```python
from build123d import *

# Parameters (mm, degrees)
F0_W      = 3
F0_H      = 11
F1_DEPTH  = 15.9
F2_W      = 6
F2_H      = 9
F3_DEPTH  = 31.001
F4_R      = 1
F5_DEPTH  = 6.9
F6_R      = 1.05
F7_DEPTH  = 4
F8_W      = 3
F8_H      = 1
F8_W_2    = 1
F8_H_2    = 3
F9_DEPTH  = 1
F10_R     = 1
F11_DEPTH = 3
F12_W     = 12
F12_H     = 8
F13_DEPTH = 3


with BuildPart() as f1:
    # F0 (on Front) → F1 (new body)
    with BuildSketch(Plane.XZ):
        with Locations((1.5, 8.5)):
            Rectangle(F0_W, F0_H)
        Polygon((3, 3), (0, 3), (0, 0), (31, 0), (31, 3), (28, 3), align=None)
        with Locations((29.5, 8.5)):
            Rectangle(F0_W, F0_H)
    extrude(amount=F1_DEPTH)

    # F2 (on face) → F3 (cut, through all)
    with BuildSketch(Plane.YZ.offset(31)):
        with Locations((-6, 9.5)):
            Rectangle(F2_W, F2_H)
    extrude(amount=-F3_DEPTH, mode=Mode.SUBTRACT)

    # F4 (on face) → F5 (cut, through all)
    with BuildSketch(Plane.XZ.offset(15.9)):
        with Locations((1.7, 8.95)):
            Circle(F4_R)
        with Locations((29.3, 8.95)):
            Circle(F4_R)
    extrude(amount=-F5_DEPTH, mode=Mode.SUBTRACT)

    # F6 (on face) → F7 (cut)
    with BuildSketch(Plane(origin=(0, 0, 0), x_dir=(-1, 0, 0), z_dir=(0, 1, 0))):
        with Locations((-26, 1.5)):
            Circle(F6_R)
        with Locations((-5, 1.5)):
            Circle(F6_R)
    extrude(amount=-F7_DEPTH, mode=Mode.SUBTRACT)

    # F8 (on face) → F9 (join)
    with BuildSketch(Plane(origin=(0, 0, 0), x_dir=(-1, 0, 0), z_dir=(0, 1, 0))):
        with Locations((-20.5, 1.5)):
            Rectangle(F8_W, F8_H)
        with Locations((-10.5, 1.5)):
            Rectangle(F8_W, F8_H)
        with Locations((-29, 9.5)):
            Rectangle(F8_W_2, F8_H_2)
        with Locations((-2, 9.5)):
            Rectangle(F8_W_2, F8_H_2)
    extrude(amount=F9_DEPTH)

    # F10 (on face) → F11 (cut)
    with BuildSketch(Plane.XY.offset(14)):
        with Locations((29.4, -1.5)):
            Circle(F10_R)
        with Locations((1.6, -1.5)):
            Circle(F10_R)
    extrude(amount=-F11_DEPTH, mode=Mode.SUBTRACT)

    # F12 (on face) → F13 (cut, through all)
    with BuildSketch(Plane.XY.offset(3)):
        with Locations((16, -7.9)):
            Rectangle(F12_W, F12_H)
    extrude(amount=-F13_DEPTH, mode=Mode.SUBTRACT)


solid = f1.part
```
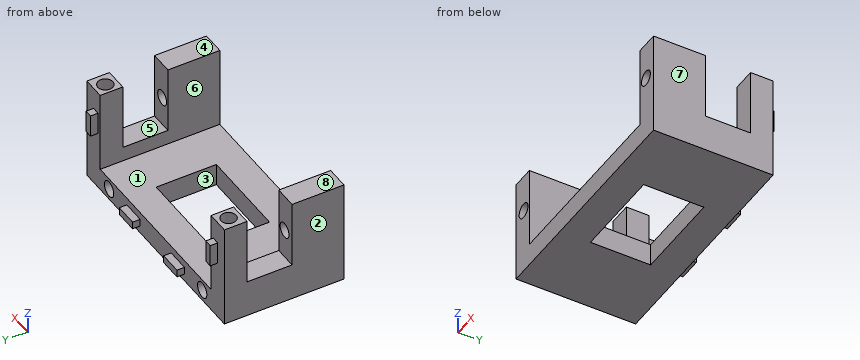
Geometry: final body of the model. Coordinates: model frame, mm. Face numbers are marked on the shaded views. A direction names the side the tool comes from. Round coordinates to 2 decimals unless told otherwise and drop trailing zeros. Order: outer loops, then holes, each group sorted by start corner. A loop starts at its lowest first (then second) coordinate and runs counter-clockwise, first axis right, second up. Notation, with made-up numbers: (77.25, 87) - (104.25, 87) arc R21 ccw to (104.25, 95) - close; hole circle Ø5 at (55.5, 2.5). An arc over 180 degrees is marked (long way). Use CSV: the item, a comma, the result in double quotes. Start each with the question number.
Q1. Mould query, pull axis X, two halves, no side actions, for the marked faces 6, 7 and 8. Classes: +X half, -X half, draft (parallel to the pull), parting line (faces both ways), or undercut.
Q2. Access query for the marked faces 1, 2, 3, 4 and 5. Directions: +Z, -Z, +X, -X, +Y, -Y. A direction counts if a zero-diameter tool reaches every point of the face in a straight line with its end or side. Return the directions, or none.
Q3. Material intervals for line 1 along Y through (x, z) = (29.4, 11.95); line 2 along Y through (x, z) = (2, 10); line 3 along Z through (x, y) = (5, -1.8), sorted ascending. Write a range as from..to.
Q4. Section query C-C (x = 10.5). Return loops of the section in (y, z).
Q5. First-contact query: pin 1 (5 mm diameter, centred on x = 20.5, y = -6, fed in from +Z); pin 2 (2.5 mm diameter, centred on x = 4.5, z = 2, fed in from +Y); pin 3 (2.5 mm diameter, centred on x = 29, y = -7, fed in from +Z). Flat tips, straight axial feed; report the tip coordinate or a pass-through.
Q6. Section query B-B (y = -4.5). Return loops of the section in (x, z).
Q7. Section query A-A (z = 7). Return loops of the section in (x, y), and give its area (3 significant figures).
Q8. Section query D-D (z = 1.5). Return loops of the section in (x, y), and give its area (3 significant figures).
Result set:
1,face 6,"undercut"
1,face 7,"+X half"
1,face 8,"draft"
2,face 1,"+Z, +Y, -Y"
2,face 2,"+Z, -Z, -X, +Y, -Y"
2,face 3,"+Z, -Z"
2,face 4,"+Z, +X, -X, +Y, -Y"
2,face 5,"+Z, +X, -X"
3,line 1,"y = -15.9..-9, -3..-2.5, -0.5..0"
3,line 2,"y = -15.9..-9, -3..1"
3,line 3,"z = 0..0.45, 2.55..3"
4,outline,"(-15.9, 0) - (-11.9, 0) - (-11.9, 3) - (-15.9, 3) - close; (-3.9, 0) - (0, 0) - (0, 1) - (1, 1) - (1, 2) - (0, 2) - (0, 3) - (-3.9, 3) - close"
5,pin 1,"stops at z = 3"
5,pin 2,"stops at y = 0"
5,pin 3,"stops at z = 5"
6,outline,"(0, 0) - (10, 0) - (10, 3) - (3, 3) - (3, 5) - (0, 5) - close; (22, 0) - (31, 0) - (31, 5) - (28, 5) - (28, 3) - (22, 3) - close"
7,outline,"(0, -15.9) - (3, -15.9) - (3, -9) - (0, -9) - close; (0, -3) - (3, -3) - (3, 0) - (0, 0) - close; (28, -15.9) - (31, -15.9) - (31, -9) - (28, -9) - close; (28, -3) - (31, -3) - (31, 0) - (28, 0) - close"
7,area,"59.4 mm2"
8,outline,"(0, -15.9) - (31, -15.9) - (31, 0) - (27.05, 0) - (27.05, -4) - (24.95, -4) - (24.95, 0) - (22, 0) - (22, 1) - (19, 1) - (19, 0) - (12, 0) - (12, 1) - (9, 1) - (9, 0) - (6.05, 0) - (6.05, -4) - (3.95, -4) - (3.95, 0) - (0, 0) - close; hole (10, -11.9) - (22, -11.9) - (22, -3.9) - (10, -3.9) - close"
8,area,"386 mm2"
